Autodesk Inventor part; units mm, degrees
ref_plane "YZ Plane" through (0, 0, 0) normal (1, 0, 0) x (0, 1, 0)
ref_plane "XZ Plane" through (0, 0, 0) normal (0, 1, 0) x (-1, 0, 0)
ref_plane "XY Plane" through (0, 0, 0) normal (0, 0, 1) x (1, 0, 0)
sketch "Sketch1" plane through (0, 0, 0) normal (0, 0, 1) x (1, 0, 0)
  line L0 (-2.425, -0.3) -> (2.425, -0.3)
  line L1 (2.425, -0.3) -> (2.425, 0.3)
  line L2 (2.425, 0.3) -> (-2.425, 0.3)
  line L3 (-2.425, 0.3) -> (-2.425, -0.3)
  line L4 (-2.425, -0.3) -> (2.425, 0.3) construction
  line L5 (2.425, -0.3) -> (-2.425, 0.3) construction
  line L6 (-3.3, -2) -> (3.3, -2)
  line L7 (3.3, -2) -> (3.3, 2)
  line L8 (3.3, 2) -> (-3.3, 2)
  line L9 (-3.3, 2) -> (-3.3, -2)
  line L10 (-3.3, -2) -> (3.3, 2) construction
  line L11 (3.3, -2) -> (-3.3, 2) construction
  line L12 (-3.3, 0) -> (3.3, 0)
  line L13 (3.3, 0) -> (3.3, 2.3)
  line L14 (3.3, 2.3) -> (-3.3, 2.3)
  line L15 (-3.3, 2.3) -> (-3.3, 0)
  line L16 (-4.3, 3.3) -> (4.3, 3.3)
  line L17 (4.3, 3.3) -> (4.3, -4)
  line L18 (4.3, -4) -> (-4.3, -4)
  line L19 (-4.3, -4) -> (-4.3, 3.3)
  point P0 (0, 0)
  point P1 (-3.3, 2)
  point P2 (3.3, 2)
  dimension "d0" = 0.6
  dimension "d1" = 4.85
  dimension "d4" = 6.6
  dimension "d6" = 2
  dimension "d9" = 1
  dimension "d10" = 1
  dimension "d11" = 1
  dimension "d12" = 2
  dimension "d20" = 2
extrude "Extrusion1" add sketch "Sketch1" along normal blind 3 contours L0 L1 L12 L7 L6 L9 L3 | L12 L9 L8 L7 L1 L2 L3 | L15 L14 L13 L8 | L16 L17 L18 L19
extrude "Extrusion2" add sketch "Sketch1" along normal blind 8
sketch "Sketch2" plane through (3.3, -2, 3) normal (-1, 0, 0) x (0, 0, 1)
  line L0 (0, 0) -> (0, 4.3)
  line L1 (0, 0) -> (5, 0)
  line L2 (5, 4.3) -> (5, 0)
  line L3 (0, 4.3) -> (5, 4.3)
  line L4 (0, 0) -> (0, 4.3)
  line L5 (0, 2.8) -> (4.1212, 4.3)
  line L6 (0, 4.3) -> (5, 4.3)
  point P0 (-3, 2)
  point P1 (0, 2.3)
  dimension "d22" = 0.5
  dimension "d23" = 70
extrude "Extrusion3" add sketch "Sketch2" along normal blind 7 contours L0 L3 L5
sketch "Sketch3" plane through (0, 0, 8) normal (0, 0, 1) x (1, 0, 0)
  line L0 (-4.3, -4) -> (4.3, -4)
  line L1 (4.3, -4) -> (4.3, 3.3)
  line L2 (4.3, 3.3) -> (-4.3, 3.3)
  line L3 (-4.3, 3.3) -> (-4.3, -4)
  line L4 (3.3, -2) -> (-3.3, -2)
  line L5 (-3.3, -2) -> (-3.3, 2.3)
  line L6 (-3.3, 2.3) -> (3.3, 2.3)
  line L7 (3.3, 2.3) -> (3.3, -2)
  line L8 (-3.3, 2.3) -> (-1.8, 2.3)
  line L9 (-1.8, 2.3) -> (-1.8, 0.8)
  line L10 (-1.8, 0.8) -> (-3.3, 0.8)
  line L11 (-3.3, 0.8) -> (-3.3, 2.3)
  line L12 (3.3, 2.3) -> (1.8, 2.3)
  line L13 (1.8, 2.3) -> (1.8, 0.8)
  line L14 (1.8, 0.8) -> (3.3, 0.8)
  line L15 (3.3, 0.8) -> (3.3, 2.3)
  point P0 (0, 0)
  point P1 (-3.3, 0.8)
  point P2 (-1.8, 2.3)
  dimension "d26" = 1.5
  dimension "d27" = 1.5
  dimension "d28" = 1.5
  dimension "d29" = 1.5
extrude "Extrusion4" add sketch "Sketch3" against normal blind 5 contours L14 L13 L6 L7 | L5 L6 L9 L10
chamfer "Chamfer2" distance 1 angle 45 1 edges at (-3.3, -2, 5.5)
chamfer "Chamfer3" distance 1 angle 45 1 edges at (3.3, -2, 5.5)
sketch "Sketch4" plane through (0, 0, 8) normal (0, 0, 1) x (1, 0, 0)
  line L0 (-2.3, -2) -> (2.3, -2)
  circle A0 centre (0, -2) radius 0.75
  point P0 (0, 0)
  dimension "d39" = 1.5
extrude "Extrusion5" cut sketch "Sketch4" against normal blind 10
fillet "Fillet2" radius 2 4 edges at (-4.3, 3.3, 4) (4.3, 3.3, 4) (4.3, -4, 4) (-4.3, -4, 4)
properties part number "Cable_tie_connector_p1_metal"
Source: CAD feature listing. Evaluate the final solid. Frame: model axes, mm. A direction names the side the tool comes from. Give positions to 0.01 mm unless a question says otherwise; leave off trailing zeros. Order: outer loops, then holes, each group sorted by start corner. A loop starts at its lowest first (then second) coordinate and runs counter-clockwise, first axis right, second up. Notation, with made-up numbers: (6.5, 76) -> (61.5, 76) arc R31 cw to (61.5, 107) -> close; hole circle Ø5 at (45, 61.25). An arc over 180 degrees is marked (long way). Write item = value, one per line.
Q1. Cut plane A-A, the plane y = -2.5. Output: boundary loops of the cut face in (x, z), and give its area (3 significant figures).
Data:
outline = (-4.24, 0) -> (-0.56, 0) -> (-0.56, 8) -> (-4.24, 8) -> close; (0.56, 0) -> (4.24, 0) -> (4.24, 8) -> (0.56, 8) -> close
area = 58.8 mm^2
Q2. Material intervals for line 1 (X direction, y = -0.5, z = 7.5); line 2 (X direction, y = -2, z = 2); line 3 (Y direction, x = -1.75, z = 2.5), sorted ascending. Write a range as from..to.
Data:
line_1 = -4.3..-3.3, 3.3..4.3
line_2 = -4.3..-0.75, 0.75..4.3
line_3 = -4..-0.3, 0.3..3.3
Q3. Cut plane C-C, the plane z = 1.25. Output: boundary loops of the cut face in (x, y) (3 decimals).
Data:
outline = (-4.3, -2) arc R2 ccw to (-2.3, -4) -> (2.3, -4) arc R2 ccw to (4.3, -2) -> (4.3, 1.3) arc R2 ccw to (2.3, 3.3) -> (-2.3, 3.3) arc R2 ccw to (-4.3, 1.3) -> close; hole (-2.425, -0.3) -> (2.425, -0.3) -> (2.425, 0.3) -> (-2.425, 0.3) -> close; hole circle Ø1.5 at (0, -2)
Q4. Set-up query: faces 5 (the face through (0, 0.3, 1)), 6 (the face through (-3.7, 2.73, 4.06)), 7 (the face through (1.8, 1, 6)). Return all of +Z, -Z, +X, -X, +Y, -Y with unobstructed straight access to the full face (end or side cutting, diameter ignored); none if empty.
Data:
face_5 = +Z, -Z
face_6 = +Z, -Z, -X, +Y
face_7 = +Z
Q5. Cut plane B-B, the plane x = 0. Output: boundary loops of the cut face in (y, z), and give its area (3 significant figures).
Data:
outline = (-4, 0) -> (-2.75, 0) -> (-2.75, 8) -> (-4, 8) -> close; (-1.25, 0) -> (-0.3, 0) -> (-0.3, 3) -> (-1.25, 3) -> close; (0.3, 0) -> (3.3, 0) -> (3.3, 8) -> (2.3, 8) -> (2.3, 7.12) -> (0.8, 3) -> (0.3, 3) -> close
area = 29.9 mm^2
Q6. Pin query (flat end, axial travel): pin 1 (0.8 mm diameter, centred on x = 0.5, y = 0, fed in from +Z); pin 2 (0.8 mm diameter, centred on y = 2, z = 6.5, fed in from -X). Return the tip coordinate at first contact, or that it passes through.
Data:
pin_1 = 3
pin_2 = -4.28
Q7. Cut plane D-D, the plane z = 5. Output: boundary loops of the cut face in (x, y), and give its area (3 significant figures).
Data:
outline = (-4.3, -2) arc R2 ccw to (-2.3, -4) -> (2.3, -4) arc R2 ccw to (4.3, -2) -> (4.3, 1.3) arc R2 ccw to (2.3, 3.3) -> (-2.3, 3.3) arc R2 ccw to (-4.3, 1.3) -> close; hole (-3.3, -1) -> (-2.3, -2) -> (-0.75, -2) arc R0.75 ccw to (0.75, -2) -> (2.3, -2) -> (3.3, -1) -> (3.3, 0.8) -> (1.8, 0.8) -> (1.8, 1.53) -> (-1.8, 1.53) -> (-1.8, 0.8) -> (-3.3, 0.8) -> close
area = 38.4 mm^2
Q8. Pull-direction query (X, two-part tool) for faces 1 (the face through (-1.8, 1, 6)), 2 (the face through (0, -4, 4)), 3 (the face through (2.8, -1.5, 5.5)), 4 (the face through (-3.73, -3.4, 4.06)); classes: released by +X, released by -X, zero draft, split by the parting line, or undercut.
Data:
face_1 = undercut
face_2 = zero draft
face_3 = undercut
face_4 = released by -X
